Source: CAD feature listing. Evaluate the final solid. Frame: model axes, mm. A direction names the side the tool comes from. Give positions to 0.01 mm unless a question says otherwise; leave off trailing zeros. Loops run counter-clockwise (first coordinate to the right, second up) from the corner with the lowest first, then second, coordinate; pieces in that order, holes last.
from build123d import *
from build123d import SkipClean  # not in build123d's __all__

# Parameters (mm, degrees)
F2_R = 0.889


with BuildPart() as f1:
    # F0 (on Front) → F1 (revolve)
    with BuildSketch(Plane.XZ):
        Polygon((8.0391, 2.7178), (8.0391, 0), (15.0368, 0), (15.0368, 2.1336), (13.8207983748, 2.1336), (12.3698, 1.1176), (9.3218, 1.1176), (9.3218, 4.4196), (8.0391, 4.4196), (8.0391, 3.7338), (8.8011, 3.7338), (8.8011, 2.7178), align=None)
    revolve(axis=Axis((0, 0, 19.8358264327), (0, 0, 1)))

    # F2 (on Front) → F3 (revolve, cut)
    with BuildSketch(Plane.XZ):
        with Locations((15.0368, 0)):
            Circle(F2_R)
    revolve(axis=Axis((0, 0, 19.8358264327), (0, 0, 1)), mode=Mode.SUBTRACT)

    # F4: F1 across plane


with BuildPart() as f1_1:
    add(f1.part, clean=False)
    with SkipClean():  # cleaning this boolean's faces spoils the solid; the shape is the same uncleaned
        add(f1.part.mirror(Plane.XY), clean=False)


solid = f1_1.part
1) Contact query for flat-ended pins moving along their axis: P1, Ø2, axis at x = 5, z = -2, coming from the -Y side (3 decimals); P2, Ø1.5, axis at x = 10, y = 10, coming from the +Z side; P3, Ø9.5, axis at x = 0, y = 0, coming from the -Z side; P4, Ø2, axis at y = 11, z = -1, coming from the -X side. Output: stop coordinate, or through.
Checks:
P1: stops at y = -14.495
P2: stops at z = 2.13
P3: passes through
P4: stops at x = -11.23
2) Pull-direction query (X, two-part tool) for faces 1 (the cylindrical face through (-3.26, -14.68, -1.52)), 2 (the flat face through (-8, -3, 4.42)), 3 (the cylindrical face through (-8.03, 0.35, -4.07)), 4 (the flat face through (-4.6, 8.3, 1.118)); classes: released by +X, released by -X, zero draft, split by the parting line, or undercut.
Checks:
face 1: split by the parting line
face 2: zero draft
face 3: undercut
face 4: undercut
3) Ray query, probe 1 along Y at (x, z) = (6.5, -1.75); probe 2 along Y at (x, z) = (0, -3.95); probe 3 along Y at (x, z) = (-6.5, -1.25). Return the intervals inside material, ascending.
Checks:
probe 1: y = -13.56 to -11.57, -6.68 to -4.73, 4.73 to 6.68, 11.57 to 13.56
probe 2: y = -9.32 to -8.04, 8.04 to 9.32
probe 3: y = -13.56 to -10.75, -6.68 to -4.73, 4.73 to 6.68, 10.75 to 13.56
4) Reachability of faces 5 (the cylindrical face through (8.89, 2.8, 2.79)), 6 (the cylindrical face through (8.89, 2.8, -2.79)), 7 (the flat face through (-8, -3, -4.42)), 8 (the cylindrical face through (8.395, 2.644, -3.219)) from +Z, -Z, +X, -X, +Y, -Y: full face, straight path, thin tool, end or side. Return the list, or none.
Checks:
face 5: +Z
face 6: -Z
face 7: -Z, +X, -X, +Y, -Y
face 8: none
5) Cut plane A-A (z = 1.5). Return loops of the section in (x, y), and give its area (3 significant figures).
Checks:
outline: circle Ø30.07 at (0, 0); circle Ø18.64 at (0, 0); hole circle Ø25.83 at (0, 0); hole circle Ø16.08 at (0, 0)
area: 256 mm2
